```python
from build123d import *

# Parameters (mm, degrees)
SKETCH1_R           = 6.1
BOSS_EXTRUDE1_DEPTH = 7.4
CUT_EXTRUDE2_DEPTH  = 7.4
CIRPATTERN1_COUNT   = 20


with BuildPart() as part:
    # Sketch1 → Boss-Extrude1 (new body)
    with BuildSketch(Plane(origin=(0, 0, 0), x_dir=(1, 0, 0), z_dir=(0, 1, 0))):
        Circle(SKETCH1_R)
    extrude(amount=BOSS_EXTRUDE1_DEPTH)

    # Sketch2 → Cut-Extrude2 (cut)
    with BuildSketch(Plane(origin=(0, 7.4, 0), x_dir=(1, 0, 0), z_dir=(0, 1, 0))):
        with BuildLine():
            Line((-38.373637849, 1.335743881), (-0.758991905, 6.05259707))
            ThreePointArc((-0.758991905, 6.05259707), (-0.648582224, 6.02243319), (-0.591589713, 5.923175892))
            ThreePointArc((-0.591589713, 5.923175892), (-0.557758828, 5.765024422), (-0.498876404, 5.614394822))
            ThreePointArc((-0.498876404, 5.614394822), (0, 5.30259707), (0.498876404, 5.614394822))
            ThreePointArc((0.498876404, 5.614394822), (0.557758828, 5.765024422), (0.591589713, 5.923175892))
            ThreePointArc((0.591589713, 5.923175892), (0.648582224, 6.02243319), (0.758991905, 6.05259707))
            Line((0.758991905, 6.05259707), (38.373637849, 1.335743881))
            Line((38.373637849, 1.335743881), (38.373637849, 77.154219029))
            Line((38.373637849, 77.154219029), (-38.373637849, 77.154219029))
            Line((-38.373637849, 77.154219029), (-38.373637849, 1.335743881))
        make_face()
    cut_extrude2 = extrude(amount=-CUT_EXTRUDE2_DEPTH, mode=Mode.SUBTRACT)

    # CirPattern1: Cut-Extrude2 ×20 about axis
    cirpattern1_axis = Axis((0, 0, 0), (0, 1, 0))
    for i in range(1, CIRPATTERN1_COUNT):
        add(cut_extrude2.rotate(cirpattern1_axis, i * 360 / CIRPATTERN1_COUNT), mode=Mode.SUBTRACT)


solid = part.part
```
Design review of the part built by this model. Coordinates are the model's own, in mm. Coordinates: 2 decimals unless noted, no trailing zeros. Order: outer loops, then holes, each group sorted by start corner. A loop starts at its lowest first (then second) coordinate and runs counter-clockwise, first axis right, second up. Notation, with made-up numbers: (57, -38.5) - (84, -38.5) arc R13 ccw to (84, -27.5) - close; hole circle Ø8 at (61, 1). An arc over 180 degrees is marked (long way). One line per question, with ' | ' between items.
Q1. Consider section B-B, the plane z = -2. Give the boundary of the cut face in (x, y).
Answer key:
outline: (-5.05, 0) - (5.05, 0) - (5.05, 7.4) - (-5.05, 7.4) - close
Q2. Consider section A-A, the plane x = 3.5. Give the boundary of the cut face in (y, z).
Answer key:
outline: (0, -4.19) - (7.4, -4.19) - (7.4, 4.19) - (0, 4.19) - close
Q3. Clearance check with flat-ended pins moving along their axes: pin 1 Ø3 at (x, y) = (-1, 2.5) entering from +Z; pin 2 Ø1.5 at (x, y) = (-3, 4.5) entering from +Z. State where each tip first meets the part, or that it passes through.
Answer key:
pin 1: stops at z = 6.05 | pin 2: stops at z = 5.54
Q4. To check wall thickness, follow line 1 along X through (y, z) = (4.5, -0.5); line 2 along Z through (x, y) = (-4.75, 1). State the ranges of each line that lie inside material, in increasing order.
Answer key:
line 1: x = -5.62 to 5.62 | line 2: z = -2.89 to 2.89
Q5. The part is to be moulded in two halves that separate along X. For faces 1 (the cylindrical face through (-1.65, 3.75, -5.04)), 2 (the cylindrical face through (-5.303, 3.752, 0.009)), 3 (the cylindrical face through (5.303, 3.752, -0.009)), say which applies: +X half, -X half, draft (parallel to the pull), parting line (faces both ways), or undercut.
Answer key:
face 1: undercut | face 2: -X half | face 3: +X half
